Can you work these out from the model? Positions are in its coordinate system, mm. Face numbers are marked on the shaded views. A direction names the side the tool comes from. Coordinates: 2 decimals unless noted, no trailing zeros. Loops run counter-clockwise (first coordinate to the right, second up) from the corner with the lowest first, then second, coordinate; pieces in that order, holes last.
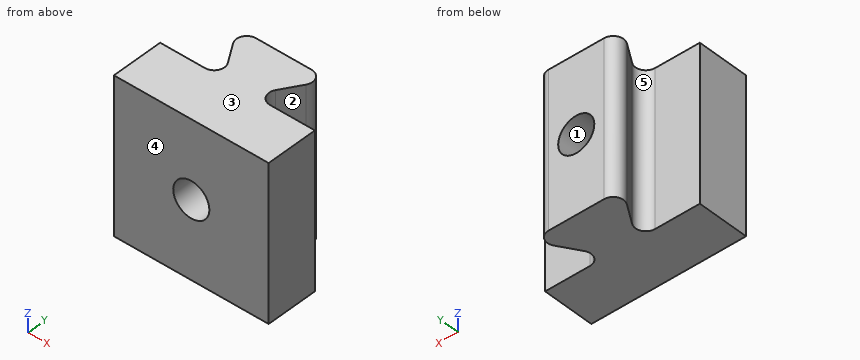
```python
from build123d import *

# Parameters (mm, degrees)
ESBO_O1_W                = 15
ESBO_O1_H                = 5
RESSALTO_EXTRUS_O1_DEPTH = 15
FILETE1_R                = 1
ESBO_O2_R                = 1.75
CORTE_EXTRUS_O1_DEPTH    = 15


with BuildPart() as part:
    # Esboço1 → Ressalto-extrusão1 (new body)
    with BuildSketch(Plane.XY):
        with Locations((0, -2.5)):
            Rectangle(ESBO_O1_W, ESBO_O1_H)
        Polygon((-4.5, 5), (-1.35, 0), (1.35, 0), (4.5, 5), align=None)
    extrude(amount=RESSALTO_EXTRUS_O1_DEPTH)

    # Filete1
    filete1_edges = [part.edges().sort_by_distance(p)[0] for p in [
        (-1.35, 0, 7.5),
        (-4.5, 5, 7.5),
        (4.5, 5, 7.5),
        (1.35, 0, 7.5),
    ]]
    fillet(filete1_edges, radius=FILETE1_R)

    # Esboço2 → Corte-extrusão1 (cut)
    with BuildSketch(Plane(origin=(0, 5, 0), x_dir=(1, 0, 0), z_dir=(0, 1, 0))):
        with Locations(Location((0, -7.5, 0), (0, 0, 270))):
            Circle(ESBO_O2_R)
    extrude(amount=-CORTE_EXTRUS_O1_DEPTH, mode=Mode.SUBTRACT)


solid = part.part
```
(1) Which directions (+Z, -Z, +X, -X, +Y, -Y) give clear straight access to the entire face, cutting with the end or side of a thin tool? Please do the marked faces 1 and 2.
Check values:
face 1: +Y, -Y
face 2: +Z, -Z, +X
(2) I want a section at D-D on z = 1.75. Write out the boundary of the cut face in (x, y).
Check values:
outline: (-7.5, -5) - (7.5, -5) - (7.5, 0) - (3.16, 0) arc R1 cw to (2.32, 1.53) - (3.53, 3.47) arc R1 ccw to (2.69, 5) - (-2.69, 5) arc R1 ccw to (-3.53, 3.47) - (-2.32, 1.53) arc R1 cw to (-3.16, 0) - (-7.5, 0) - close
(3) If we mould it in two halves opening along Y, with no side actions, what happens to the marked faces 3, 4 and 5? For each: released by +Y, released by -Y, zero draft, split by the parting line, or undercut.
Check values:
face 3: zero draft
face 4: released by -Y
face 5: undercut
(4) I want a section at C-C on x = 0. Write out the boundary of the cut face in (y, z), then the cut area to 3 significant figures.
Check values:
outline: (-5, 0) - (5, 0) - (5, 5.75) - (-5, 5.75) - close; (-5, 9.25) - (5, 9.25) - (5, 15) - (-5, 15) - close
area: 115 mm2
(5) I want a section at A-A on z = 7.5. Write out the boundary of the cut face in (x, y), then the cut area to 4 significant figures.
Check values:
outline: (-7.5, -5) - (-1.75, -5) - (-1.75, 5) - (-2.69, 5) arc R1 ccw to (-3.53, 3.47) - (-2.32, 1.53) arc R1 cw to (-3.16, 0) - (-7.5, 0) - close; (1.75, -5) - (7.5, -5) - (7.5, 0) - (3.16, 0) arc R1 cw to (2.32, 1.53) - (3.53, 3.47) arc R1 ccw to (2.69, 5) - (1.75, 5) - close
area: 69.25 mm2
(6) I'm going to push flat-ended pins straight in: pin 1 (1.3 mm diameter, centred on x = -6, z = 8, fed in from +Y); pin 2 (2 mm diameter, centred on y = 2.5, z = 2.5, fed in from +X). Where does each tip first touch, or does it pass through?
Check values:
pin 1: stops at y = 0
pin 2: stops at x = 3.55
(7) I want a section at B-B on y = -2. Write out the boundary of the cut face in (x, z), then the cut area to 3 significant figures.
Check values:
outline: (-7.5, 0) - (7.5, 0) - (7.5, 15) - (-7.5, 15) - close; hole circle Ø3.5 at (0, 7.5)
area: 215 mm2
(8) If I drill on probe 1 along X at (y, z) = (-0.5, 7.5); probe 2 along Y at (x, z) = (6.25, 5); probe 3 along Y at (x, z) = (3, 14), over which ranges is the centre line in solid material (lowest first)?
Check values:
probe 1: x = -7.5 to -1.75, 1.75 to 7.5
probe 2: y = -5 to 0
probe 3: y = -5 to 0.01, 2.62 to 4.95
